```python
from build123d import *

# Parameters (mm, degrees)
F0_R     = 3.175
F1_DEPTH = 3


with BuildPart() as f1:
    # F0 (on Top) → F1 (new body, symmetric)
    with BuildSketch(Plane.XY):
        with BuildLine():
            Line((-97.928558, -28.24017), (-21.728558, -28.24017))
            Line((-21.728558, -28.24017), (-21.728558, 40.65983))
            ThreePointArc((-21.728558, 40.65983), (-27.586423, 54.801966), (-41.728558, 60.65983))
            Line((-41.728558, 60.65983), (-77.928558, 60.65983))
            ThreePointArc((-77.928558, 60.65983), (-92.070694, 54.801966), (-97.928558, 40.65983))
            Line((-97.928558, 40.65983), (-97.928558, -28.24017))
        make_face()
        with Locations((-59.828558, -20.06517)):
            Circle(F0_R, mode=Mode.SUBTRACT)
    extrude(amount=F1_DEPTH, both=True)


solid = f1.part
```
The listing builds one solid part. Answer for the finished solid, in the listing's coordinates (mm). Coordinates: 2 decimals unless noted, no trailing zeros. Write each loop counter-clockwise with the first axis right and the second up, starting at its lowest first coordinate (ties: lowest second). Pieces come first, ordered by that corner, then holes.
Q1. Find the intervals of material crossed by line 1 along X through (y, z) = (-22, -0.6); line 2 along Y through (x, z) = (-57, -1); line 3 along Y through (x, z) = (-36.5, -0.8), in increasing order.
Returned:
line 1: x = -97.93 to -62.35, -57.31 to -21.73
line 2: y = -28.24 to -21.51, -18.62 to 60.66
line 3: y = -28.24 to 59.96
Q2. Section C-C, the plane y = 49.5 is taken. Write down the section's boundary in (x, z).
Returned:
outline: (-95.87, -3) - (-23.79, -3) - (-23.79, 3) - (-95.87, 3) - close
Q3. Section B-B, the plane x = -60 is taken. Write down the section's boundary in (y, z), then the cut area to 3 significant figures.
Returned:
outline: (-28.24, -3) - (-23.24, -3) - (-23.24, 3) - (-28.24, 3) - close; (-16.89, -3) - (60.66, -3) - (60.66, 3) - (-16.89, 3) - close
area: 495 mm2
Q4. Section A-A, the plane z = -0.4 is taken. Write down the section's boundary in (x, y) (3 decimals).
Returned:
outline: (-97.929, -28.24) - (-21.729, -28.24) - (-21.729, 40.66) arc R20 ccw to (-41.729, 60.66) - (-77.929, 60.66) arc R20 ccw to (-97.929, 40.66) - close; hole circle Ø6.35 at (-59.829, -20.065)
